```python
from build123d import *

# Parameters (mm, degrees)
EXTRUDE_1_DEPTH = 7
CHAMFER_1_SIZE  = 1
CHAMFER_1_SIZE2 = 1.732050808


with BuildPart() as part:
    # Эскиз1 → Бобышка-Вытянуть1 (new body)
    with BuildSketch(Plane.XY):
        Polygon((0, 0), (0, 1.9), (2, 1.9), (2, 5), (-7, 5), (-7, 0), align=None)
    extrude(amount=EXTRUDE_1_DEPTH)

    # Эскиз4 → Отверстие с зазором M31 (revolve, cut)
    with BuildSketch(Plane(origin=(-3, 5, 4), x_dir=(0, 0, 1), z_dir=(1, 0, 0))):
        Polygon((0, 0), (0, 5), (1.725, 5), (1.7, 4.975), (1.7, 0.025), (1.725, 0), align=None)
    revolve(axis=Axis((-3, 11.35, 4), (0, -1, 0)), mode=Mode.SUBTRACT)

    # Фаска1
    chamfer_1_edges = [part.edges().sort_by_distance(p)[0] for p in [
        (-7, 2.5, 0),
    ]]
    chamfer_1_side = [part.faces().sort_by_distance(p)[0] for p in [
        (-7, 2.5, 3.5),
    ]]
    chamfer(chamfer_1_edges, length=CHAMFER_1_SIZE, length2=CHAMFER_1_SIZE2, reference=chamfer_1_side[0])


solid = part.part
```
Model file for the job. Use its own axes, mm. A direction names the side the tool comes from. Coordinates: 2 decimals unless noted, no trailing zeros. Loops run counter-clockwise (first coordinate to the right, second up) from the corner with the lowest first, then second, coordinate; pieces in that order, holes last. Notation, with made-up numbers: (-21.75, 17) - (6.25, 17) arc R27 ccw to (6.25, 51) - close; hole circle Ø7 at (75.5, 43.25). An arc over 180 degrees is marked (long way). Answer as a JSON object with one key per item and string values. Group by question number.
(1) Flat gauge pin, fed straight in: pin 1 (2.5 mm diameter, centred on x = -3, z = 4, fed in from +Y). Where does the tip first touch, or does it go through?
(2) Cut at A-A (x = -3). Give the cut face in (y, z) (3 decimals), then the cut area to 3 significant figures.
(3) Cut at C-C (y = 3). Give the cut face in (x, z), then the cut area to 3 significant figures.
(4) Tool access for faces 4 (the face through (1, 1.9, 3)), 5 (the face through (-6.12, 2.53, 0.49)): list every direction of +Z, -Z, +X, -X, +Y, -Y with a clear straight run to the whole face (end or side of a thin tool).
(5) Cut at D-D (z = 6.25). Give the cut face in (x, y), then the cut area to 3 significant figures.
(6) Cut at B-B (z = 4). Give the cut face in (x, y) (3 decimals), then the cut area to 3 significant figures.
(7) Two-plate mould, pull along X, no slides. Class faces 1 (the face through (-7, 3, 4)), 2 (the face through (-4.433, 2.535, 4.914)), 3 (the face through (-2, 3, 0)): released by +X, released by -X, zero draft, split by the parting line, or undercut.
(8) Probe line 1 along X through (y, z) = (2.75, 4); line 2 along Z through (x, y) = (-3, 3.7); line 3 along Z through (x, y) = (-2.25, 4.85). List the from-to ranges inside material, lowest first.
Geometry says:
{
 "1": {"pin 1": "passes through"},
 "2": {"outline": "(0, 0) - (5, 0) - (5, 2.275) - (4.975, 2.3) - (0.025, 2.3) - (0, 2.275) - close; (0, 5.725) - (0.025, 5.7) - (4.975, 5.7) - (5, 5.725) - (5, 7) - (0, 7) - close", "area": "18.0 mm^2"},
 "3": {"outline": "(-7, 1) - (-5.27, 0) - (2, 0) - (2, 7) - (-7, 7) - close; hole circle Ø3.4 at (-3, 4)", "area": "53.1 mm^2"},
 "4": {"face 4": "+Z, -Z, +X, -Y", "face 5": "-Z, -X, +Y, -Y"},
 "5": {"outline": "(-7, 0) - (0, 0) - (0, 1.9) - (2, 1.9) - (2, 5) - (-7, 5) - close", "area": "41.2 mm^2"},
 "6": {"outline": "(-7, 0) - (-4.725, 0) - (-4.7, 0.025) - (-4.7, 4.975) - (-4.725, 5) - (-7, 5) - close; (-1.3, 0.025) - (-1.275, 0) - (0, 0) - (0, 1.9) - (2, 1.9) - (2, 5) - (-1.275, 5) - (-1.3, 4.975) - close", "area": "24.2 mm^2"},
 "7": {"face 1": "released by -X", "face 2": "undercut", "face 3": "zero draft"},
 "8": {"line 1": "x = -7 to -4.7, -1.3 to 2", "line 2": "z = 0 to 2.3, 5.7 to 7", "line 3": "z = 0 to 2.47, 5.53 to 7"}
}
